The model under review builds one solid part; all positions refer to its coordinate system, in mm. Coordinates: 2 decimals unless noted, no trailing zeros. Write each loop counter-clockwise with the first axis right and the second up, starting at its lowest first coordinate (ties: lowest second). Pieces come first, ordered by that corner, then holes. Notation, with made-up numbers: (77.5, 11) - (110.5, 11) arc R20 ccw to (110.5, 25) - close; hole circle Ø6 at (3.5, 70). An arc over 180 degrees is marked (long way). Put each result on its own line as item: value. Start each with the question number.
Item 1: Consider section B-B on z = 68. Give the boundary of the cut face in (x, y).
Item 2: To check wall thickness, follow L1, parallel to Y at x = 0, z = 22; L2, parallel to X at y = -0.5, z = 15.5; L3, parallel to Y at x = 2.5, z = 18.5. State the ranges of each line that lie inside material, in increasing order. Write a range as [from, to].
Item 3: Consider section C-C on x = -1.5. Give the boundary of the cut face in (y, z), then the cut area to 3 significant figures.
Item 4: Consider section A-A on y = 0. Give the boundary of the cut face in (x, z), then the cut area to 3 significant figures.
Item 5: Mouldability with a two-part tool opening along X and no side actions: class faces 1 (the face through (17.439, -3, 50)), 2 (the face through (-15.63, 14.49, 51.51)), 3 (the face through (4, 8, 0)), 4 (the face through (-5.95, 5.46, 50.09)) as pulls with the +X half, pulls with the -X half, needs draft (parallel to the pull), parting line crosses it, or undercut.
Item 6: Consider section D-D on x = 14. Give the boundary of the cut face in (y, z).
```python
from build123d import *

# Parameters (mm, degrees)
F0_W     = 34.877166
F0_H     = 32.801156
F0_R     = 8.075164
F1_DEPTH = 101.6
F2_R     = 6.35


with BuildPart() as f1:
    # F0 (on Top) → F1 (new body)
    with BuildSketch(Plane.XY):
        Rectangle(F0_W, F0_H)
        Circle(F0_R, mode=Mode.SUBTRACT)
    extrude(amount=F1_DEPTH)

    # F2
    f2_edges = [f1.edges().sort_by_distance(p)[0] for p in [
        (-17.438583, 16.400578, 50.8),
        (17.438583, 16.400578, 50.8),
    ]]
    fillet(f2_edges, radius=F2_R)


solid = f1.part
```
Report:
1. outline: (-17.44, -16.4) - (17.44, -16.4) - (17.44, 10.05) arc R6.35 ccw to (11.09, 16.4) - (-11.09, 16.4) arc R6.35 ccw to (-17.44, 10.05) - close; hole circle Ø16.15 at (0, 0)
2. L1: [-16.4, -8.08], [8.08, 16.4]
2. L2: [-17.44, -8.06], [8.06, 17.44]
2. L3: [-16.4, -7.68], [7.68, 16.4]
3. outline: (-16.4, 0) - (-7.93, 0) - (-7.93, 101.6) - (-16.4, 101.6) - close; (7.93, 0) - (16.4, 0) - (16.4, 101.6) - (7.93, 101.6) - close
3. area: 1,720 mm²
4. outline: (-17.44, 0) - (-8.08, 0) - (-8.08, 101.6) - (-17.44, 101.6) - close; (8.08, 0) - (17.44, 0) - (17.44, 101.6) - (8.08, 101.6) - close
4. area: 1,900 mm²
5. face 1: pulls with the +X half
5. face 2: pulls with the -X half
5. face 3: needs draft
5. face 4: undercut
6. outline: (-16.4, 0) - (15.69, 0) - (15.69, 101.6) - (-16.4, 101.6) - close
